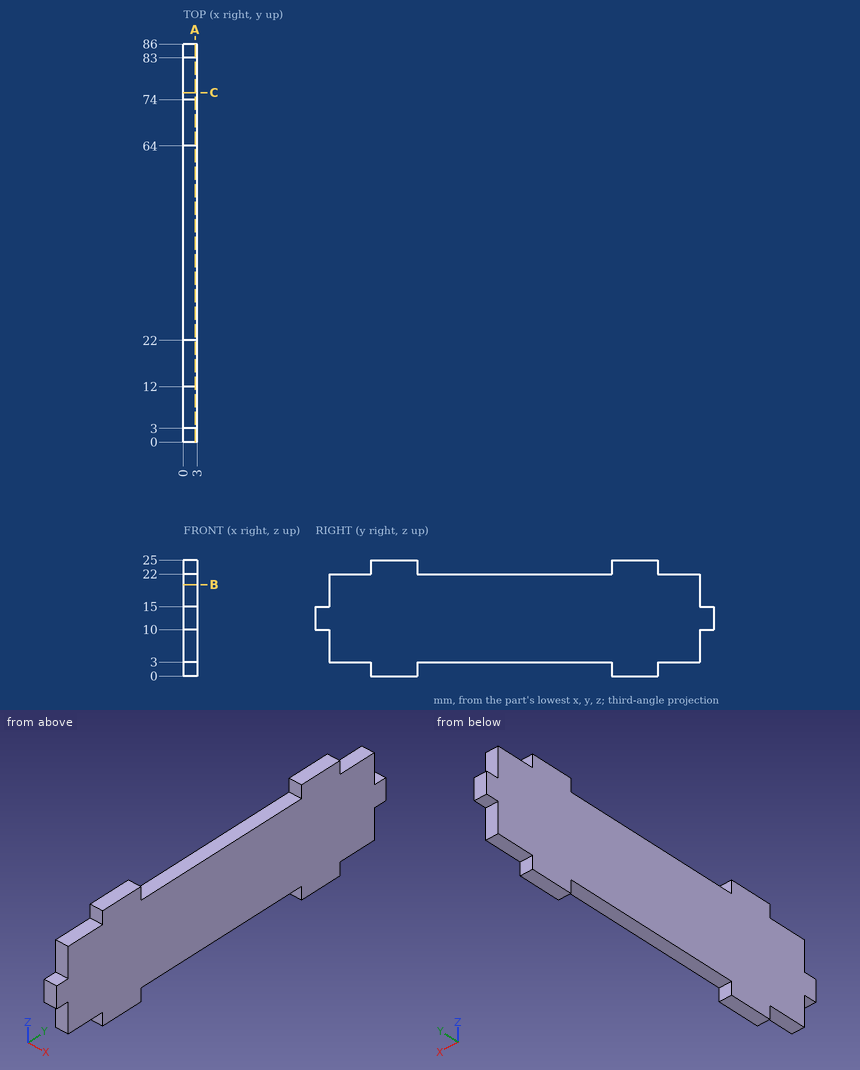
Can you work these out from the drawing? Everything is in mm from the part's minimum corner. Give positions to 0.01 mm unless a question says otherwise; leave off trailing zeros. Loops run counter-clockwise (first coordinate to the right, second up) from the corner with the lowest first, then second, coordinate; pieces in that order, holes last. Notation, with made-up numbers: (-2.75, 81) -> (48.25, 81) arc R13 cw to (48.25, 90) -> close; hole circle Ø7 at (-38.75, 84.25). An arc over 180 degrees is marked (long way). Return JSON: item names as keys, results as strings.
Q1. I want a section at B-B, the plane z = 19.75. List the corners of the cut face in (x, y) for me, then the cut area to 3 significant figures.
Checks:
{"outline": "(0, 3) -> (3, 3) -> (3, 83) -> (0, 83) -> close", "area": "240 mm2"}
Q2. I want a section at C-C, the plane y = 75.5. List the corners of the cut face in (x, z) for me.
Checks:
{"outline": "(0, 3) -> (3, 3) -> (3, 22) -> (0, 22) -> close"}
Q3. I need wall thicknesses on probe 1 along Z at (x, y) = (1.7, 39); probe 2 along Y at (x, z) = (0.2, 8.5); probe 3 along Y at (x, z) = (2.9, 23.5). Which ranges of each line are inside material? Lowest first, please.
Checks:
{"probe 1": "z = 3 to 22", "probe 2": "y = 3 to 83", "probe 3": "y = 12 to 22, 64 to 74"}
Q4. For pin 1 Ø0.9 at (x, y) = (1, 42) entering from +Z; pin 2 Ø0.9 at (x, y) = (1, 47) entering from -Z; pin 3 Ø0.9 at (x, z) = (1, 7.5) entering from +Y, each with a flat end and sliding along its axis, tell me the tip position at first contact or that it passes through.
Checks:
{"pin 1": "stops at z = 22", "pin 2": "stops at z = 3", "pin 3": "stops at y = 83"}
Q5. I want a section at A-A, the plane x = 2.55. List the corners of the cut face in (y, z) for me, then the cut area to 3 significant figures.
Checks:
{"outline": "(0, 10) -> (3, 10) -> (3, 3) -> (12, 3) -> (12, 0) -> (22, 0) -> (22, 3) -> (64, 3) -> (64, 0) -> (74, 0) -> (74, 3) -> (83, 3) -> (83, 10) -> (86, 10) -> (86, 15) -> (83, 15) -> (83, 22) -> (74, 22) -> (74, 25) -> (64, 25) -> (64, 22) -> (22, 22) -> (22, 25) -> (12, 25) -> (12, 22) -> (3, 22) -> (3, 15) -> (0, 15) -> close", "area": "1,670 mm2"}
